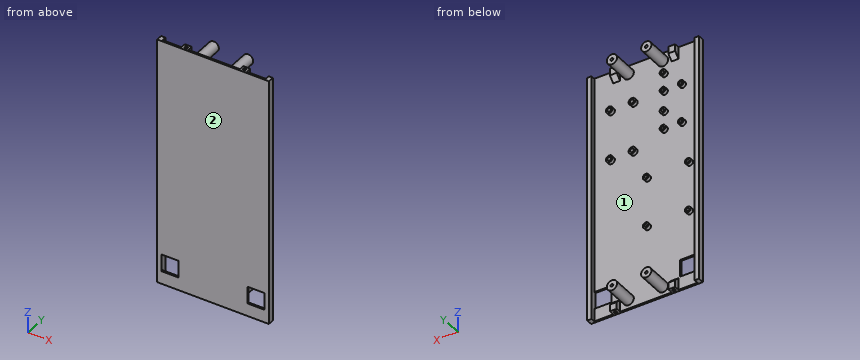
Autodesk Inventor part; units mm, degrees
ref_plane "YZ Plane" through (0, 0, 0) normal (1, 0, 0) x (0, 1, 0)
ref_plane "XZ Plane" through (0, 0, 0) normal (0, 1, 0) x (-1, 0, 0)
ref_plane "XY Plane" through (0, 0, 0) normal (0, 0, 1) x (1, 0, 0)
sketch "Sketch1" plane through (0, 0, 0) normal (0, 1, 0) x (-1, 0, 0)
  line L0 (65, -145) -> (-65, -145)
  line L1 (-65, -145) -> (-65, 145)
  line L2 (-65, 145) -> (65, 145)
  line L3 (65, 145) -> (65, -145)
  line L4 (65, 0) -> (-65, 0) construction
  line L5 (0, -145) -> (0, 145) construction
  point P0 (0, 0)
  point P1 (0, 0)
  dimension "d0" = 130
  dimension "d1" = 290
extrude "Extrusion1" add sketch "Sketch1" along normal blind 2
sketch "Sketch2" plane through (0, 0, 0) normal (0, -1, 0) x (1, 0, 0)
  line L0 (65, -145) -> (-65, -145) construction
  line L1 (0, -145) -> (0, 145) construction
  line L2 (-65, 145) -> (65, 145) construction
  line L3 (65, 145) -> (65, -145) construction
  line L4 (65, 0) -> (-65, 0) construction
  line L5 (-65, -145) -> (-65, 145) construction
  line L6 (-38, -145) -> (-30, -145)
  line L7 (-30, -145) -> (-30, -131)
  line L8 (-30, -131) -> (-38, -131)
  line L9 (-38, -131) -> (-38, -145)
  line L10 (38, -145) -> (30, -145)
  line L11 (30, -145) -> (30, -131)
  line L12 (30, -131) -> (38, -131)
  line L13 (38, -131) -> (38, -145)
  line L14 (-38, 145) -> (-30, 145)
  line L15 (-30, 145) -> (-30, 131)
  line L16 (-30, 131) -> (-38, 131)
  line L17 (-38, 131) -> (-38, 145)
  line L18 (30, 145) -> (30, 131)
  line L19 (38, 131) -> (38, 145)
  line L20 (30, 131) -> (38, 131)
  line L21 (38, 145) -> (30, 145)
  point P0 (0, 0)
  dimension "d4" = 8
  dimension "d5" = 14
  dimension "d6" = 30
extrude "Extrusion2" add sketch "Sketch2" against normal blind 8
chamfer "Chamfer1" distance 6 angle 45 4 edges at (-34, 8, 131) (34, 8, 131) (-34, 8, -131) (34, 8, -131)
sketch "Sketch3" plane through (65, 0, -145) normal (0, 0, -1) x (-1, 0, 0)
  line L0 (65, 0) -> (65, 2) construction
  line L1 (35, 2) -> (95, 2) construction
  circle A0 centre (31, 4) radius 1.75
  line L2 (27, 8) -> (35, 8)
  line L3 (35, 2) -> (35, 8)
  circle A1 centre (99, 4) radius 1.75
  dimension "d12" = 3.5
  dimension "d13" = 4
  dimension "d14" = 4
extrude "Extrusion3" cut sketch "Sketch3" against normal blind 6
sketch "Sketch4" plane through (-65, 0, 145) normal (0, 0, 1) x (1, 0, 0)
  circle A0 centre (99, 4) radius 1.75
  circle A1 centre (31, 4) radius 1.75
  point P0 (65, 0)
extrude "Extrusion4" cut sketch "Sketch4" against normal blind 6
sketch "Sketch5" plane through (0, 2, 0) normal (0, 1, 0) x (1, 0, 0)
  line L0 (-60, 130) -> (-40, 130)
  line L1 (-40, 130) -> (-40, 110)
  line L2 (-40, 110) -> (-60, 110)
  line L3 (-60, 110) -> (-60, 130)
  line L4 (-38, 145) -> (-65, 145)
  line L5 (-65, 145) -> (-65, -145)
  line L6 (-65, 145) -> (65, 145) construction
  line L7 (0, 145) -> (0, -145) construction
  line L8 (-30, -145) -> (30, -145) construction
  line L9 (60, 130) -> (40, 130)
  line L10 (40, 130) -> (40, 110)
  line L11 (40, 110) -> (60, 110)
  line L12 (60, 110) -> (60, 130)
  point P0 (0, 0)
  dimension "d19" = 20
  dimension "d20" = 20
  dimension "d21" = 15
  dimension "d22" = 5
extrude "Extrusion5" cut sketch "Sketch5" against normal up to next
sketch "Sketch6" plane through (0, 2, 0) normal (0, 1, 0) x (1, 0, 0)
  line L0 (-51.5, -1.5) -> (-2.5, -1.5) construction
  line L1 (-2.5, -1.5) -> (-2.5, 56.5) construction
  line L2 (-2.5, 56.5) -> (-51.5, 56.5) construction
  line L3 (-51.5, 56.5) -> (-51.5, -1.5) construction
  line L4 (65, -145) -> (-65, -145) construction
  line L5 (-65, 145) -> (65, 145) construction
  line L6 (-27, -1.5) -> (-27, 56.5) construction
  line L7 (-40, 110) -> (-60, 110) construction
  line L8 (-55, -5) -> (1, -5) construction
  line L9 (1, -5) -> (1, 80) construction
  line L10 (1, 80) -> (-55, 80) construction
  line L11 (-55, 80) -> (-55, -5) construction
  circle A0 centre (-2.5, -1.5) radius 1.75
  circle A1 centre (-51.5, -1.5) radius 1.75
  circle A2 centre (-51.5, 56.5) radius 1.75
  circle A3 centre (-2.5, 56.5) radius 1.75
  circle A4 centre (-2.5, -1.5) radius 3.5
  circle A5 centre (-2.5, 56.5) radius 3.5
  circle A6 centre (-51.5, -1.5) radius 3.5
  circle A7 centre (-51.5, 56.5) radius 3.5
  line L12 (-65, 145) -> (-65, -145)
  point P0 (0, 0)
  dimension "d25" = 49
  dimension "d26" = 58
  dimension "d28" = 56
  dimension "d29" = 85
  dimension "d30" = 3.5
  dimension "d31" = 3.5
  dimension "d32" = 30
  dimension "d33" = 3.5
  dimension "d34" = 3.5
  dimension "d35" = 3.5
  dimension "d36" = 3.5
  dimension "d79" = 10
extrude "Extrusion6" add sketch "Sketch6" along normal blind 4
sketch "Sketch7" plane through (0, 2, 0) normal (0, 1, 0) x (1, 0, 0)
  line L0 (-45.4, -121) -> (-20, -121) construction
  line L1 (-20, -121) -> (-20, -50.2) construction
  line L2 (-20, -50.2) -> (-45.4, -50.2) construction
  line L3 (-45.4, -50.2) -> (-45.4, -121) construction
  line L4 (-30, -145) -> (30, -145) construction
  line L5 (30, 145) -> (-30, 145) construction
  line L6 (-38, -131) -> (-30, -131) construction
  line L7 (-20, -121) -> (-45.4, -121) construction
  line L8 (-45.4, -121) -> (-45.4, -95.6) construction
  line L9 (-45.4, -95.6) -> (-20, -95.6) construction
  line L10 (-20, -95.6) -> (-20, -121) construction
  line L11 (-45.4, -75.6) -> (-20, -75.6) construction
  line L12 (-20, -75.6) -> (-20, -50.2) construction
  line L13 (-20, -50.2) -> (-45.4, -50.2) construction
  line L14 (-45.4, -50.2) -> (-45.4, -75.6) construction
  line L15 (-20, -108.3) -> (-45.4, -108.3) construction
  line L16 (-43.241, -118.841) -> (-22.159, -118.841) construction
  line L17 (-22.159, -118.841) -> (-22.159, -97.759) construction
  line L18 (-22.159, -97.759) -> (-43.241, -97.759) construction
  line L19 (-43.241, -97.759) -> (-43.241, -118.841) construction
  line L20 (-43.241, -108.3) -> (-22.159, -108.3) construction
  line L21 (-32.7, -118.841) -> (-32.7, -97.759) construction
  circle A0 centre (-43.241, -97.759) radius 1.75
  circle A1 centre (-43.241, -97.759) radius 3.5
  circle A2 centre (-22.159, -97.759) radius 1.75
  circle A3 centre (-22.159, -97.759) radius 3.5
  circle A4 centre (-22.159, -118.841) radius 1.75
  circle A5 centre (-22.159, -118.841) radius 3.5
  line L22 (-43.241, -73.441) -> (-22.159, -73.441) construction
  line L23 (-22.159, -73.441) -> (-22.159, -52.359) construction
  line L24 (-22.159, -52.359) -> (-43.241, -52.359) construction
  line L25 (-43.241, -52.359) -> (-43.241, -73.441) construction
  line L26 (-43.241, -62.9) -> (-22.159, -62.9) construction
  line L27 (-32.7, -73.441) -> (-32.7, -52.359) construction
  circle A6 centre (-43.241, -52.359) radius 3.5
  circle A7 centre (-43.241, -52.359) radius 1.75
  circle A8 centre (-22.159, -52.359) radius 3.5
  circle A9 centre (-22.159, -52.359) radius 1.75
  circle A10 centre (-22.159, -73.441) radius 3.5
  circle A11 centre (-22.159, -73.441) radius 1.75
  line L28 (-45.4, -62.9) -> (-20, -62.9) construction
  line L29 (65, -145) -> (-65, -145) construction
  line L30 (0, -145) -> (0, 145) construction
  point P0 (0, 0)
  point P1 (-32.7, -108.3)
  point P2 (-32.7, -62.9)
  dimension "d39" = 25.4
  dimension "d40" = 10
  dimension "d41" = 25.4
  dimension "d42" = 25.4
  dimension "d57" = 21.082
  dimension "d58" = 21.082
  dimension "d61" = 3.5
  dimension "d62" = 7
  dimension "d63" = 3.5
  dimension "d64" = 7
  dimension "d65" = 3.5
  dimension "d66" = 7
  dimension "d67" = 21.082
  dimension "d68" = 21.082
  dimension "d71" = 3.5
  dimension "d72" = 7
  dimension "d73" = 3.5
  dimension "d74" = 7
  dimension "d76" = 7
  dimension "d91" = 20
  dimension "d92" = 20
extrude "Extrusion7" add sketch "Sketch7" along normal blind 4
sketch "Sketch8" plane through (0, 2, 0) normal (0, 1, 0) x (1, 0, 0)
  line L0 (-65, 145) -> (65, 145) construction
  line L1 (0, 145) -> (0, -145) construction
  line L2 (-30, -145) -> (30, -145) construction
  line L3 (-65, -145) -> (-65, 145) construction
  line L4 (-65, 0) -> (65, 0) construction
  line L5 (65, 145) -> (65, -145) construction
  circle A0 centre (-20, 135) radius 6
  circle A1 centre (20, 135) radius 6
  circle A2 centre (-20, -135) radius 6
  circle A3 centre (20, -135) radius 6
  point P0 (0, 0)
  dimension "d80" = 12
  dimension "d81" = 10
  dimension "d82" = 40
extrude "Extrusion8" add sketch "Sketch8" along normal blind 30
sketch "Sketch9" plane through (-20, 32, 135) normal (0, 1, 0) x (1, 0, 0)
  circle A0 centre (0, 0) radius 6
  circle A1 centre (40, 0) radius 6
  circle A2 centre (0, 270) radius 6
  circle A3 centre (40, 270) radius 6
  line L0 (-45, 280) -> (-45, -10) construction
  line L1 (-45, 135) -> (85, 135) construction
  line L2 (85, -10) -> (85, 280) construction
  line L3 (-45, 280) -> (85, 280) construction
  line L4 (20, 280) -> (20, -10) construction
  line L5 (-10, -10) -> (50, -10) construction
  circle A4 centre (0, 270) radius 1.625
  circle A5 centre (40, 270) radius 1.625
  circle A6 centre (0, 0) radius 1.625
  circle A7 centre (40, 0) radius 1.625
  point P0 (20, 135)
  dimension "d85" = 3.25
extrude "Extrusion9" cut sketch "Sketch9" against normal blind 10 contours A4 | A5 | A6 | A7
sketch "Sketch10" plane through (0, 2, 0) normal (0, 1, 0) x (1, 0, 0)
  line L0 (65, -145) -> (-65, -145) construction
  line L1 (0, -145) -> (0, 145) construction
  line L2 (-65, 145) -> (65, 145) construction
  line L3 (65, -145) -> (60, -145)
  line L4 (60, -145) -> (60, 145)
  line L5 (60, 145) -> (65, 145)
  line L6 (65, 145) -> (65, -145)
  line L7 (-65, -145) -> (-60, -145)
  line L8 (-60, -145) -> (-60, 145)
  line L9 (-60, 145) -> (-65, 145)
  line L10 (-65, 145) -> (-65, -145)
  point P0 (0, 0)
  point P1 (-65, 145)
extrude "Extrusion10" add sketch "Sketch10" along normal blind 5
sketch "Sketch11" plane through (0, 2, 0) normal (0, 1, 0) x (1, 0, 0)
  line L0 (13.5, -97.75) -> (40, -97.75) construction
  line L1 (40, -97.75) -> (40, -39.25) construction
  line L2 (40, -39.25) -> (13.5, -39.25) construction
  line L3 (13.5, -39.25) -> (13.5, -97.75) construction
  line L4 (60, 145) -> (60, -145) construction
  line L5 (3.75, -101) -> (49.75, -101) construction
  line L6 (49.75, -101) -> (49.75, -36) construction
  line L7 (49.75, -36) -> (3.75, -36) construction
  line L8 (3.75, -36) -> (3.75, -101) construction
  line L9 (26.75, -97.75) -> (26.75, -39.25) construction
  line L10 (13.5, -68.5) -> (40, -68.5) construction
  line L11 (30, -131) -> (38, -131) construction
  circle A0 centre (13.5, -97.75) radius 2.25
  circle A1 centre (13.5, -97.75) radius 4
  circle A2 centre (13.5, -39.25) radius 2.25
  circle A3 centre (13.5, -39.25) radius 4
  circle A4 centre (40, -39.25) radius 2.25
  circle A5 centre (40, -39.25) radius 4
  circle A6 centre (40, -97.75) radius 2.25
  circle A7 centre (40, -97.75) radius 4
  point P0 (0, 0)
  dimension "d93" = 26.5
  dimension "d94" = 58.5
  dimension "d95" = 20
  dimension "d96" = 46
  dimension "d97" = 65
  dimension "d98" = 30
  dimension "d99" = 4.5
  dimension "d100" = 8
  dimension "d101" = 4.5
  dimension "d102" = 8
  dimension "d103" = 4.5
  dimension "d104" = 8
  dimension "d105" = 4.5
  dimension "d106" = 8
extrude "Extrusion11" add sketch "Sketch11" along normal blind 4
properties part number "raspi_board_tray"
For this review, take the finished solid that the model builds, in its own axes (mm). Face numbers are marked on the shaded views. Give positions to 0.01 mm unless a question says otherwise; leave off trailing zeros. Loops run counter-clockwise (first coordinate to the right, second up) from the corner with the lowest first, then second, coordinate; pieces in that order, holes last. Notation, with made-up numbers: M 84,9.5 L 95,9.5 A30 ccw 95,47.5 Z; hole C 54.5,8 d2. An arc over 180 degrees is marked long. Put each result on its own line as item: value. Start each with the question number.
(1) The part is to be moulded in two halves that separate along Z. For the marked faces 1 and 2, say which applies: +Z half, -Z half, draft (parallel to the pull), parting line (faces both ways), or undercut.
(2) Wall thickness on L1, parallel to X at y = 3.8, z = 1.5; L2, parallel to Z at x = -20, y = 27.75 (3 decimals); L3, parallel to Z at x = 40, y = 4.9: over which ranges is each line inside the solid? List them lowest first.
(3) For pin 1 (3 mm diameter, centred on x = -22.159, z = 73.441, fed in from +Y); pin 2 (2 mm diameter, centred on x = -53, z = -56.5, fed in from +Y); pin 3 (12 mm diameter, centred on x = -11, y = 24.5, fed in from +Z), all flat-tipped, find the tip position at first contact; note any pin that passes through.
(4) Add section A-A, the plane y = 25. Write out the cut boundary in (x, z) (3 decimals).
(5) Add section B-B, the plane z = -30. Write out the cut boundary in (x, y), then the cut area to 3 significant figures.
Result:
1. face 1: undercut
1. face 2: draft
2. L1: x = -65 to -60, -55 to -53.25, -49.75 to -48, -6 to -4.25, -0.75 to 1, 60 to 65
2. L2: z = -141 to -136.625, -133.375 to -129, 129 to 133.375, 136.625 to 141
2. L3: z = 35.25 to 37, 41.5 to 43.25, 93.75 to 95.5, 100 to 101.75
3. pin 1: stops at y = 2
3. pin 2: stops at y = 6
3. pin 3: stops at z = 140.2
4. outline: C -20,-135 d12; C -20,135 d12; C 20,-135 d12; C 20,135 d12; hole C -20,-135 d3.25; hole C -20,135 d3.25; hole C 20,-135 d3.25; hole C 20,135 d3.25
5. outline: M -65,0 L 65,0 L 65,7 L 60,7 L 60,2 L -60,2 L -60,7 L -65,7 Z
5. area: 310 mm^2
